Geometry check sheet. Reference: the model listing, model coordinates, mm. A direction names the side the tool comes from. Coordinates: 2 decimals unless noted, no trailing zeros. Write each loop counter-clockwise with the first axis right and the second up, starting at its lowest first coordinate (ties: lowest second). Pieces come first, ordered by that corner, then holes. Notation, with made-up numbers: (-20.5, 19) -> (6.5, 19) arc R8 cw to (6.5, 30) -> close; hole circle Ø5 at (76.5, -5). An arc over 180 degrees is marked (long way). Use a Markdown table: item, result.
```python
from build123d import *

# Parameters (mm, degrees)
SKETCH1_R           = 14
BOSS_EXTRUDE1_DEPTH = 10
SKETCH2_R           = 2.25
CUT_EXTRUDE1_DEPTH  = 5
SKETCH3_R           = 5
CUT_EXTRUDE2_DEPTH  = 1.8
SKETCH4_W           = 10
SKETCH4_H           = 10
BOSS_EXTRUDE2_DEPTH = 8
SKETCH6_W           = 8
SKETCH6_H           = 9.912865289
BOSS_EXTRUDE3_DEPTH = 20
CUT_EXTRUDE3_DEPTH  = 30
BOSS_EXTRUDE4_DEPTH = 80


with BuildPart() as part:
    # Sketch1 → Boss-Extrude1 (new body)
    with BuildSketch(Plane.XY):
        Circle(SKETCH1_R)
    extrude(amount=BOSS_EXTRUDE1_DEPTH)

    # Sketch2 → Cut-Extrude1 (cut)
    with BuildSketch(Plane(origin=(0, 0, 0), x_dir=(-1, 0, 0), z_dir=(0, 0, -1))):
        Circle(SKETCH2_R)
    extrude(amount=-CUT_EXTRUDE1_DEPTH, mode=Mode.SUBTRACT)

    # Sketch3 → Cut-Extrude2 (cut)
    with BuildSketch(Plane(origin=(0, 0, 0), x_dir=(-1, 0, 0), z_dir=(0, 0, -1))):
        Circle(SKETCH3_R)
    extrude(amount=-CUT_EXTRUDE2_DEPTH, mode=Mode.SUBTRACT)

    # Sketch4 → Boss-Extrude2 (add)
    with BuildSketch(Plane.XY.offset(10)):
        Rectangle(SKETCH4_W, SKETCH4_H)
    extrude(amount=BOSS_EXTRUDE2_DEPTH)

    # Sketch6 → Boss-Extrude3 (add)
    with BuildSketch(Plane.ZY.offset(5)):
        with Locations((14, -0.043567356)):
            Rectangle(SKETCH6_W, SKETCH6_H)
    extrude(amount=BOSS_EXTRUDE3_DEPTH)

    # Sketch7 → Cut-Extrude3 (cut)
    with BuildSketch(Plane(origin=(5, 0, 0), x_dir=(0, 0, -1), z_dir=(1, 0, 0))):
        with BuildLine():
            Line((-18, 5), (-18, -5))
            Line((-18, -5), (-14, -5))
            ThreePointArc((-14, -5), (-14.330383596, 0), (-14, 5))
            Line((-14, 5), (-18, 5))
        make_face()
    extrude(amount=-CUT_EXTRUDE3_DEPTH, mode=Mode.SUBTRACT)

    # Sketch8 → Boss-Extrude4 (add)
    with BuildSketch(Plane.ZY.offset(25)):
        with BuildLine():
            Line((-36.180314108, 14.403585903), (13.83114902, 14.403585903))
            ThreePointArc((13.83114902, 14.403585903), (14.156322075, -2.818810644), (14, -20.043567356))
            Line((14, -20.043567356), (-36, -20.043567356))
            ThreePointArc((-36, -20.043567356), (-36.369728572, -2.821454147), (-36.180314108, 14.403585903))
        make_face()
    extrude(amount=BOSS_EXTRUDE4_DEPTH)


solid = part.part
```
Item 1: Tool access check on faces 4 (the cylindrical face through (0.29, 2.23, 3.38)), 5 (the flat face through (-15, 4.913, 12)), 6 (the cylindrical face through (-64.44, -2.578, 14.155)), 7 (the cylindrical face through (-64.44, -3.06, -36.37)). Record the directions out of +Z, -Z, +X, -X, +Y, -Y that give a thin tool (end or side, any length) a straight path to the whole face; none if there is none.
Answer block:
| item | result |
|---|---|
| face 4 | -Z |
| face 5 | +Z, +Y |
| face 6 | +Z, -X |
| face 7 | -Z, +X, -X |
Item 2: Section check A-A on y = 7. Record the boundary of the cut face in (x, z).
Answer block:
| item | result |
|---|---|
| outline | (-105, -36.33) -> (-25, -36.33) -> (-25, 14.03) -> (-105, 14.03) -> close; (-12.12, 0) -> (12.12, 0) -> (12.12, 10) -> (-12.12, 10) -> close |
Item 3: Mould release check, pull along Y, two halves, no side actions. Record for faces 1 (the cylindrical face through (12.932, -5.362, 4.93)), 2 (the flat face through (-2.2, -1, 1.8)), 3 (the flat face through (-64, 14.404, -12)): +Y half, -Y half, draft (parallel to the pull), parting line (faces both ways), or undercut.
Answer block:
| item | result |
|---|---|
| face 1 | parting line |
| face 2 | undercut |
| face 3 | +Y half |
Item 4: Section check D-D on z = -14. Record the boundary of the cut face in (x, y), then the cut area to 3 significant figures.
Answer block:
| item | result |
|---|---|
| outline | (-105, -20.04) -> (-25, -20.04) -> (-25, 14.4) -> (-105, 14.4) -> close |
| area | 2,760 mm^2 |
Item 5: Thickness scan on L1, parallel to Y at x = 0, z = 2.5; L2, parallel to X at y = -14, z = -30.5; L3, parallel to X at y = -2.5, z = 1. Record the ranges inside material, lowest first. Write a range as [from, to].
Answer block:
| item | result |
|---|---|
| L1 | y = [-14, -2.25], [2.25, 14] |
| L2 | x = [-105, -25] |
| L3 | x = [-105, -25], [-13.77, -4.33], [4.33, 13.77] |
Item 6: Section check B-B on x = 0. Record the boundary of the cut face in (y, z), then the cut area to 3 significant figures.
Answer block:
| item | result |
|---|---|
| outline | (-14, 0) -> (-5, 0) -> (-5, 1.8) -> (-2.25, 1.8) -> (-2.25, 5) -> (2.25, 5) -> (2.25, 1.8) -> (5, 1.8) -> (5, 0) -> (14, 0) -> (14, 10) -> (5, 10) -> (5, 14) arc R38 ccw to (-5, 14) -> (-5, 10) -> (-14, 10) -> close |
| area | 290 mm^2 |
Item 7: Depth check by flat-ended pin: P1, Ø3.5, axis at x = 0, y = 0, coming from the +Z side; P2, Ø3, axis at x = 0, y = 1, coming from the -Z side; P3, Ø10, axis at x = -13.5, y = -15.5, coming from the -Z side; P4, Ø1.2, axis at x = -17, z = 11.5, coming from the +Y side. Enter the tip coordinate at first touch or a pass-through.
Answer block:
| item | result |
|---|---|
| P1 | stops at z = 14.33 |
| P2 | stops at z = 1.8 |
| P3 | passes through |
| P4 | stops at y = 4.91 |
Item 8: Section check C-C on y = 0. Record the boundary of the cut face in (x, z), then the cut area to 3 significant figures.
Answer block:
| item | result |
|---|---|
| outline | (-105, -36.38) -> (-25, -36.38) -> (-25, 10) -> (-14, 10) -> (-14, 0) -> (-5, 0) -> (-5, 1.8) -> (-2.25, 1.8) -> (-2.25, 5) -> (2.25, 5) -> (2.25, 1.8) -> (5, 1.8) -> (5, 0) -> (14, 0) -> (14, 10) -> (5, 10) -> (5, 14.33) -> (-25, 14.33) -> (-25, 14.14) -> (-105, 14.14) -> close |
| area | 4,420 mm^2 |
